The listing builds one solid part. Answer for the finished solid, in the listing's coordinates (mm). Coordinates: 2 decimals unless noted, no trailing zeros. Loops run counter-clockwise (first coordinate to the right, second up) from the corner with the lowest first, then second, coordinate; pieces in that order, holes last. Notation, with made-up numbers: (58, 30.5) -> (89, 30.5) arc R16 ccw to (89, 48.5) -> close; hole circle Ø1 at (85.5, 70.5). An arc over 180 degrees is marked (long way). Answer in a Markdown table with one row per item.
```python
from build123d import *

# Parameters (mm, degrees)
CROQUIS1_R              = 1.75
CROQUIS1_R_2            = 2
SALIENTE_EXTRUIR1_DEPTH = 3


with BuildPart() as part:
    # Croquis1 → Saliente-Extruir1 (new body)
    with BuildSketch(Plane(origin=(0, 0, 0), x_dir=(0, 0, -1), z_dir=(1, 0, 0))):
        with BuildLine():
            ThreePointArc((0.225128417, -51.483442404), (6.890995422, -54.628621427), (9.447658726, -47.71563316))
            ThreePointArc((9.447658726, -47.71563316), (3.98237778, -26.07129422), (10.967929509, -4.868729021))
            ThreePointArc((10.967929509, -4.868729021), (11.945328824, -1.144167506), (11.692718634, 2.698208841))
            ThreePointArc((11.692718634, 2.698208841), (-2.21241308, 75.268149846), (4.858559991, 148.819155042))
            ThreePointArc((4.858559991, 148.819155042), (1.234772605, 154.845135355), (-4.831112169, 151.288547713))
            ThreePointArc((-4.831112169, 151.288547713), (-16.879167042, 49.539087028), (0.225128417, -51.483442404))
        make_face()
        with Locations((5, -50)):
            Circle(CROQUIS1_R, mode=Mode.SUBTRACT)
        with Locations((0, 150)):
            Circle(CROQUIS1_R, mode=Mode.SUBTRACT)
        Circle(CROQUIS1_R, mode=Mode.SUBTRACT)
        with Locations((-7, 35)):
            Circle(CROQUIS1_R_2, mode=Mode.SUBTRACT)
        with Locations((-7, 115)):
            Circle(CROQUIS1_R_2, mode=Mode.SUBTRACT)
    extrude(amount=SALIENTE_EXTRUIR1_DEPTH)


solid = part.part
```
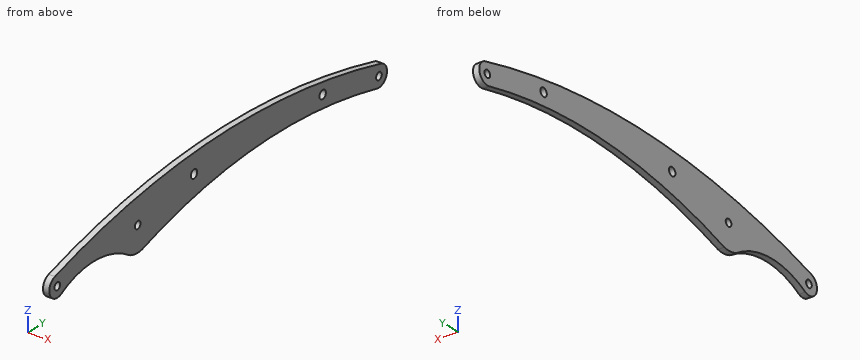
Item 1: Find the intervals of material crossed by probe 1 along Z at (x, y) = (0.95, 150); probe 2 along Z at (x, y) = (2.3, -4.5); probe 3 along Z at (x, y) = (2.75, 88), in increasing order.
Findings below:
| item | result |
|---|---|
| probe 1 | z = -5 to -1.75, 1.75 to 5.17 |
| probe 2 | z = -11.12 to 11.43 |
| probe 3 | z = 2.5 to 15.78 |
Item 2: A cutting plane is placed at C-C, the plane z = 7. Determine the outline of the cut face in (x, y), plus the area to 3 significant figures.
Findings below:
| item | result |
|---|---|
| outline | (0, -25.71) -> (3, -25.71) -> (3, 33) -> (0, 33) -> close; (0, 37) -> (3, 37) -> (3, 113) -> (0, 113) -> close; (0, 117) -> (3, 117) -> (3, 142.74) -> (0, 142.74) -> close |
| area | 481 mm2 |
Item 3: A cutting plane is placed at D-D, the plane y = 115. Determine the outline of the cut face in (x, z), plus the area to 3 significant figures.
Findings below:
| item | result |
|---|---|
| outline | (0, 1.03) -> (3, 1.03) -> (3, 5) -> (0, 5) -> close; (0, 9) -> (3, 9) -> (3, 12.53) -> (0, 12.53) -> close |
| area | 22.5 mm2 |
Item 4: A cutting plane is placed at B-B, the plane x = 1.25. Determine the outline of the cut face in (y, z), plus the area to 3 significant figures.
Findings below:
| item | result |
|---|---|
| outline | (-51.48, -0.23) arc R5 ccw (long way) to (-47.72, -9.45) arc R40 cw to (-4.87, -10.97) arc R12 ccw to (2.7, -11.69) arc R260 cw to (148.82, -4.86) arc R5 ccw to (151.29, 4.83) arc R360 ccw to start; hole circle Ø3.5 at (-50, -5); hole circle Ø3.5 at (0, 0); hole circle Ø4 at (35, 7); hole circle Ø4 at (115, 7); hole circle Ø3.5 at (150, 0) |
| area | 3,020 mm2 |
Item 5: A cutting plane is placed at A-A, the plane y = 0. Determine the outline of the cut face in (x, z), plus the area to 3 significant figures.
Findings below:
| item | result |
|---|---|
| outline | (0, -12) -> (3, -12) -> (3, -1.75) -> (0, -1.75) -> close; (0, 1.75) -> (3, 1.75) -> (3, 12.2) -> (0, 12.2) -> close |
| area | 62.1 mm2 |
